Build history of the part. All positions in model axes, mm. Face numbers are marked on the shaded views. A direction names the side the tool comes from. Round coordinates to 2 decimals unless told otherwise and drop trailing zeros. Write each loop counter-clockwise with the first axis right and the second up, starting at its lowest first coordinate (ties: lowest second). Pieces come first, ordered by that corner, then holes. Notation, with made-up numbers: (35.25, -12.75) -> (47.25, -12.75) arc R24 ccw to (47.25, 9.25) -> close; hole circle Ø5 at (55, 68). An arc over 180 degrees is marked (long way). Answer as CSV lines item,"result".
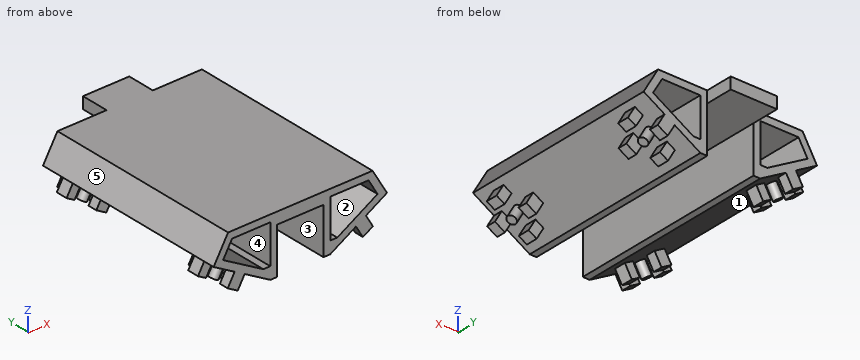
from build123d import *

# Parameters (mm, degrees)
BOSS_EXTRU_1_DEPTH          = 87
ENL_V_MAT_EXTRU_1_REACH     = 99.981
BOSS_EXTRU_2_DEPTH          = 87
ESQUISSE3_R                 = 1.9
ESQUISSE3_W                 = 5
ESQUISSE3_H                 = 4
ESQUISSE3_W_2               = 4
ESQUISSE3_H_2               = 5
BOSS_EXTRU_3_DEPTH          = 6
SYM_TRIE3_COPY_1_SKETCH_R   = 1.9
SYM_TRIE3_COPY_1_SKETCH_W   = 5
SYM_TRIE3_COPY_1_SKETCH_H   = 4
SYM_TRIE3_COPY_1_SKETCH_W_2 = 4
SYM_TRIE3_COPY_1_SKETCH_H_2 = 5
SYM_TRIE3_COPY_1_DEPTH      = 6
ESQUISSE5_W                 = 20
ESQUISSE5_H                 = 5
BOSS_EXTRU_4_DEPTH          = 12


with BuildPart() as part:
    # Esquisse1 → Boss.-Extru.1 (new body)
    with BuildSketch(Plane(origin=(0, 0, 0), x_dir=(1, 0, 0), z_dir=(0, 1, 0))):
        Polygon((-31.25, 0), (31.25, 0), (37.5, 10.825317547), (12.948729811, 25), (10, 25), (10, 5), (-10, 5), (-10, 25), (-12.948729811, 25), (-37.5, 10.825317547), align=None)
    extrude(amount=BOSS_EXTRU_1_DEPTH)

    # Esquisse2 → Enlèv. mat.-Extru.1 (cut, up to next)
    with BuildSketch(Plane(origin=(0, 87, 0), x_dir=(1, 0, 0), z_dir=(0, 1, 0)), mode=Mode.PRIVATE) as enl_v_mat_extru_1_sk1:
        Polygon((-36, 8.227241336), (-16, 19.77424672), (-13, 19.77424672), (-13, 0), (-31.25, 0), align=None)
    enl_v_mat_extru_1_tool1 = extrude(enl_v_mat_extru_1_sk1.sketch, amount=-ENL_V_MAT_EXTRU_1_REACH, mode=Mode.PRIVATE) & part.part
    enl_v_mat_extru_1 = enl_v_mat_extru_1_tool1.solids().sort_by_distance((-22.148909, 87, -8.14347))[0]
    add(enl_v_mat_extru_1, mode=Mode.SUBTRACT)

    # Symétrie1: Enlèv. mat.-Extru.1 across plane
    add(enl_v_mat_extru_1.mirror(Plane(origin=(0, 0, 0), x_dir=(0, 0, 1), z_dir=(1, 0, 0))), mode=Mode.SUBTRACT)

    # Esquisse4 → Boss.-Extru.2 (add)
    with BuildSketch(Plane(origin=(0, 0, 0), x_dir=(1, 0, 0), z_dir=(0, 1, 0))):
        Polygon((-37.5, 10.825317547), (-31.25, 0), (31.25, 0), (37.5, 10.825317547), (34.901923789, 12.325317547), (29.517949192, 3), (-29.517949192, 3), (-34.901923789, 12.325317547), align=None)
    extrude(amount=BOSS_EXTRU_2_DEPTH)

    # Esquisse3 → Boss.-Extru.3 (add)
    with BuildSketch(Plane(origin=(-14.0625, 0, -24.356964481), x_dir=(0.8660254037844396, 0, -0.4999999999999984), z_dir=(0.49999999999999833, 0, 0.8660254037844395))):
        with Locations((-14.063293868, 77)):
            Circle(ESQUISSE3_R)
        with Locations((-14.063293868, 85)):
            Rectangle(ESQUISSE3_W, ESQUISSE3_H)
        with Locations((-22.063293868, 77)):
            Rectangle(ESQUISSE3_W_2, ESQUISSE3_H_2)
        with Locations((-6.063293868, 77)):
            Rectangle(ESQUISSE3_W_2, ESQUISSE3_H_2)
        with Locations((-14.063293868, 69)):
            Rectangle(ESQUISSE3_W, ESQUISSE3_H)
    boss_extru_3 = extrude(amount=-BOSS_EXTRU_3_DEPTH)

    # Symétrie2: Boss.-Extru.3 across plane
    add(boss_extru_3.mirror(Plane.ZX.offset(43.5)))

    # Symétrie3: Boss.-Extru.3 across plane
    add(boss_extru_3.mirror(Plane(origin=(0, 0, 0), x_dir=(0, 0, 1), z_dir=(1, 0, 0))))

    # Symétrie3 copy 1 sketch → Symétrie3 copy 1 (add)
    with BuildSketch(Plane(origin=(14.0625, 87, -24.356964481), x_dir=(-0.8660254037844396, 0, -0.4999999999999984), z_dir=(-0.49999999999999833, 0, 0.8660254037844395))):
        with Locations((-14.063293868, 77)):
            Circle(SYM_TRIE3_COPY_1_SKETCH_R)
        with Locations((-14.063293868, 85)):
            Rectangle(SYM_TRIE3_COPY_1_SKETCH_W, SYM_TRIE3_COPY_1_SKETCH_H)
        with Locations((-22.063293868, 77)):
            Rectangle(SYM_TRIE3_COPY_1_SKETCH_W_2, SYM_TRIE3_COPY_1_SKETCH_H_2)
        with Locations((-6.063293868, 77)):
            Rectangle(SYM_TRIE3_COPY_1_SKETCH_W_2, SYM_TRIE3_COPY_1_SKETCH_H_2)
        with Locations((-14.063293868, 69)):
            Rectangle(SYM_TRIE3_COPY_1_SKETCH_W, SYM_TRIE3_COPY_1_SKETCH_H)
    extrude(amount=-SYM_TRIE3_COPY_1_DEPTH)

    # Esquisse5 → Boss.-Extru.4 (add)
    with BuildSketch(Plane(origin=(0, 87, 0), x_dir=(1, 0, 0), z_dir=(0, 1, 0))):
        with Locations((0, 2.5)):
            Rectangle(ESQUISSE5_W, ESQUISSE5_H)
    extrude(amount=BOSS_EXTRU_4_DEPTH)


solid = part.part
1. Cut at D-D, the plane x = 19.5. Write the cut outline in (y, z).
Results found:
outline,"(0, -21.22) -> (7.5, -21.22) -> (7.5, -25.65) -> (12.5, -25.65) -> (12.5, -21.22) -> (74.5, -21.22) -> (74.5, -25.65) -> (79.5, -25.65) -> (79.5, -21.22) -> (87, -21.22) -> (87, -17.75) -> (0, -17.75) -> close; (0, -3) -> (87, -3) -> (87, 0) -> (0, 0) -> close"
2. Cut at A-A, the plane y = 58. Write the cut outline in (x, z).
Results found:
outline,"(-37.5, -10.83) -> (-12.95, -25) -> (-10, -25) -> (-10, -5) -> (10, -5) -> (10, -25) -> (12.95, -25) -> (37.5, -10.83) -> (31.25, 0) -> (-31.25, 0) -> close; hole (-33.4, -9.73) -> (-16, -19.77) -> (-13, -19.77) -> (-13, -3) -> (-29.52, -3) -> close; hole (13, -19.77) -> (16, -19.77) -> (33.4, -9.73) -> (29.52, -3) -> (13, -3) -> close"
3. Mould opens along Y. For the marked faces 1 and 2 say: +Y half, -Y half, draft (parallel to the pull), parting line (faces both ways), or undercut.
Results found:
face 1,"undercut"
face 2,"draft"
4. Probe line 1 along X through (y, z) = (14.5, -23.25); line 2 along Y through (x, z) = (-30.5, -20.5); line 3 along X through (y, z) = (16.5, -12). List the from-to ranges inside material, lowest first.
Results found:
line 1,"x = -15.98 to -10, 10 to 15.98"
line 2,"y = 0 to 4, 16 to 20, 67 to 71, 83 to 87"
line 3,"x = -35.47 to -29.47, -13 to -10, 10 to 13, 29.47 to 35.47"
5. Cut at C-C, the plane z = -8. Write the cut outline in (x, y), then the cut area to 3 significant figures.
Results found:
outline,"(-35.87, 0) -> (-32.4, 0) -> (-32.4, 87) -> (-35.87, 87) -> close; (-13, 0) -> (-10, 0) -> (-10, 87) -> (-13, 87) -> close; (10, 0) -> (13, 0) -> (13, 87) -> (10, 87) -> close; (32.4, 0) -> (35.87, 0) -> (35.87, 87) -> (32.4, 87) -> close"
area,"1,120 mm2"
6. Cut at B-B, the plane x = -19. Write the cut outline in (y, z).
Results found:
outline,"(0, -21.51) -> (7.5, -21.51) -> (7.5, -24.78) -> (12.5, -24.78) -> (12.5, -21.51) -> (74.5, -21.51) -> (74.5, -24.78) -> (79.5, -24.78) -> (79.5, -21.51) -> (87, -21.51) -> (87, -18.04) -> (0, -18.04) -> close; (0, -3) -> (87, -3) -> (87, 0) -> (0, 0) -> close"
7. Which spindle directions (+Z, -Z, +X, -X, +Y, -Y) get a long thin tool onto all of the face, cutting with end or side? Do the marked faces 3, 4 and 5. Say none if no direction does.
Results found:
face 3,"-Z, +Y, -Y"
face 4,"+Y, -Y"
face 5,"+Z, -X, +Y, -Y"
8. Drop flat-ended pins along their axis: pin 1 Ø7 at (x, z) = (21, -23.5) entering from +Y; pin 2 Ø4 at (x, z) = (-6.5, -16.5) entering from -Y; pin 3 Ø1.5 at (y, z) = (76.5, -3.5) entering from -X; pin 4 Ø6 at (x, y) = (-14, 26.5) entering from -Z. Give the stop position or say it passes through.
Results found:
pin 1,"stops at y = 87"
pin 2,"passes through"
pin 3,"stops at x = -33.7"
pin 4,"stops at z = -25"
